from build123d import *

# Parameters (mm, degrees)
BOSS_EXTRU_1_DEPTH      = 7.9
ESQUISSE2_R             = 1.6
ESQUISSE2_R_2           = 4
ENL_V_MAT_EXTRU_1_DEPTH = 8.9
CONG_1_R                = 2


with BuildPart() as part:
    # Esquisse1 → Boss.-Extru.1 (new body)
    with BuildSketch(Plane(origin=(0, 0, 0), x_dir=(0, 0, -1), z_dir=(1, 0, 0))):
        with BuildLine():
            Line((37.960924758, 1.984416578), (37.960924758, 6.984416578))
            Line((37.960924758, 6.984416578), (29.410924758, 6.984416578))
            Line((29.410924758, 6.984416578), (29.410924758, 12.984416578))
            Line((29.410924758, 12.984416578), (187.175507503, 124.984416578))
            Line((187.175507503, 124.984416578), (194.410924758, 124.984416578))
            ThreePointArc((194.410924758, 124.984416578), (202.410924758, 116.984416578), (194.410924758, 108.984416578))
            Line((194.410924758, 108.984416578), (187.175507503, 108.984416578))
            Line((187.175507503, 108.984416578), (64.410924758, 12.984416578))
            Line((64.410924758, 12.984416578), (64.410924758, 6.984416578))
            Line((64.410924758, 6.984416578), (53.860924758, 6.984416578))
            Line((53.860924758, 6.984416578), (53.860924758, 1.984416578))
            Line((53.860924758, 1.984416578), (37.960924758, 1.984416578))
        make_face()
    extrude(amount=BOSS_EXTRU_1_DEPTH)

    # Esquisse2 → Enlèv. mat.-Extru.1 (cut, through all)
    with BuildSketch(Plane(origin=(7.9, 0, 0), x_dir=(0, 0, -1), z_dir=(1, 0, 0))):
        with Locations((45.910924758, 11.184416578)):
            Circle(ESQUISSE2_R)
        with Locations((194.410924758, 117.118890011)):
            Circle(ESQUISSE2_R_2)
    extrude(amount=-ENL_V_MAT_EXTRU_1_DEPTH, mode=Mode.SUBTRACT)

    # Congé1
    cong_1_edges = [part.edges().sort_by_distance(p)[0] for p in [
        (3.95, 12.984416578, -64.410924758),
        (3.95, 108.984416578, -187.175507503),
        (3.95, 124.984416578, -187.175507503),
        (3.95, 12.984416578, -29.410924758),
    ]]
    fillet(cong_1_edges, radius=CONG_1_R)


solid = part.part
CAD build for the part. Positions are in the model's coordinates, mm. A direction names the side the tool comes from. Coordinates: 2 decimals unless noted, no trailing zeros. Loops run counter-clockwise (first coordinate to the right, second up) from the corner with the lowest first, then second, coordinate; pieces in that order, holes last. Notation, with made-up numbers: (29.25, 45) - (56.25, 45) arc R14 cw to (56.25, 50) - close; hole circle Ø5 at (-24.75, -26). An arc over 180 degrees is marked (long way). Use one line per item in the form item = value. Start each with the question number.
1) Band-saw the part on A-A (x = 3.5). Give the cut face in (y, z).
2) Band-saw the part on C-C (z = -50). Give the cut face in (x, y).
3) Tool access for faces 1 (the face through (4, 6.984, -34)), 2 (the face through (4, 6.984, -59)), 3 (the face through (7.9, 59, -110)): list every direction of +Z, -Z, +X, -X, +Y, -Y with a clear straight run to the whole face (end or side of a thin tool).
4) Two-plate mould, pull along Y, no slides. Class faces 4 (the face through (4.01, 12.77, -45.7)), 5 (the face through (3.89, 68.32, -107.36)), 6 (the face through (4, 9, -29.411)): +Y half, -Y half, draft (parallel to the pull), parting line (faces both ways), or undercut.
5) Drill centre lines: L1, parallel to Z at x = 4.5, y = 12; L2, parallel to Z at x = 4.25, y = 116.5; L3, parallel to Y at x = 6.25, z = -91. Where is each one in solid material? Low to high. Write a range as from..to.
6) Flat gauge pins, fed straight in: pin 1 (4 mm diameter, centred on x = 2, z = -127.5, fed in from +Y); pin 2 (2.5 mm diameter, centred on x = 5.5, z = -35, fed in from -Y); pin 3 (2 mm diameter, centred on x = 6.5, z = -128.5, fed in from -Y); pin 4 (10.5 mm diameter, centred on y = 117.12, z = -194.41, fed in from +X). Where does each tip first touch, or does it go through?
7) Band-saw the part on B-B (y = 20.5). Give the cut face in (x, z), and give its area (3 significant figures).
Check values:
q1.outline = (1.98, -53.86) - (6.98, -53.86) - (6.98, -64.41) - (12.01, -64.41) arc R2 cw to (13.58, -65.18) - (108.56, -186.63) arc R2 cw to (108.98, -187.86) - (108.98, -194.41) arc R8 ccw to (124.98, -194.41) - (124.98, -187.81) arc R2 ccw to (124.62, -186.66) - (13.58, -30.25) arc R2 ccw to (11.95, -29.41) - (6.98, -29.41) - (6.98, -37.96) - (1.98, -37.96) - close; hole circle Ø3.2 at (11.18, -45.91); hole circle Ø8 at (117.12, -194.41)
q2.outline = (0, 1.98) - (7.9, 1.98) - (7.9, 27.6) - (0, 27.6) - close
q3.face_1 = +Z, +X, -X, -Y
q3.face_2 = -Z, +X, -X, -Y
q3.face_3 = +Z, -Z, +X, +Y, -Y
q4.face_4 = undercut
q4.face_5 = +Y half
q4.face_6 = draft
q5.L1 = -64.41..-47.29, -44.53..-29.41
q5.L2 = -202.4..-198.36, -190.46..-175.22
q5.L3 = 33.78..56.71
q6.pin_1 = 84.04
q6.pin_2 = 6.98
q6.pin_3 = 62.32
q6.pin_4 = 7.9
q7.outline = (0, -74.02) - (7.9, -74.02) - (7.9, -40) - (0, -40) - close
q7.area = 269 mm2
